from build123d import *

# Parameters (mm, degrees)
SKETCH_1_W                  = 720
SKETCH_1_H                  = 300
EXTRUDE_1_DEPTH             = 6
SKETCH_2_R                  = 30
CUT_EXTRUDE_1_DEPTH         = 13
SKETCH_5_R                  = 22.5
CUT_EXTRUDE_2_DEPTH         = 13
HOLE_WIZARD_M6_1_D          = 5
HOLE_WIZARD_13_0_13_1_D     = 13
HOLE_WIZARD_4_D             = 6.6
HOLE_WIZARD_4_CBORE_D       = 11
HOLE_WIZARD_4_CBORE_DEPTH   = 6.8
HOLE_WIZARD_11_0_11_1_D     = 11
HOLE_WIZARD_11_0_11_2_D     = 11
SKETCH_29_W                 = 170
SKETCH_29_H                 = 170
CUT_EXTRUDE_5_DEPTH         = 13
CUT_EXTRUDE_6_DEPTH         = 13
HOLE_WIZARD_M5_3_D          = 4.2
SKETCH_32_R                 = 28
CUT_EXTRUDE_7_DEPTH         = 13
HOLE_WIZARD_4_2_D           = 6.6
HOLE_WIZARD_4_2_CBORE_D     = 11
HOLE_WIZARD_4_2_CBORE_DEPTH = 6.8
HOLE_WIZARD_M6_2_D          = 5
SKETCH_38_W                 = 100
SKETCH_38_H                 = 110
CUT_EXTRUDE_8_DEPTH         = 13
HOLE_WIZARD_M6_3_D          = 5
FILLET_1_R                  = 10


with BuildPart() as part:
    # 草图1 → 凸台-拉伸1 (new body, symmetric)
    with BuildSketch(Plane.XY):
        Rectangle(SKETCH_1_W, SKETCH_1_H)
    extrude(amount=EXTRUDE_1_DEPTH, both=True)

    # 草图2 → 切除-拉伸1 (cut, through all)
    with BuildSketch(Plane.XY.offset(6)):
        with Locations((45, 0)):
            Circle(SKETCH_2_R)
    extrude(amount=-CUT_EXTRUDE_1_DEPTH, mode=Mode.SUBTRACT)

    # 草图5 → 切除-拉伸2 (cut, through all)
    with BuildSketch(Plane.XY.offset(6)):
        with Locations((-130, 87.5)):
            Circle(SKETCH_5_R)
        with Locations((-130, -87.5)):
            Circle(SKETCH_5_R)
        with Locations((220, -87.5)):
            Circle(SKETCH_5_R)
        with Locations((220, 87.5)):
            Circle(SKETCH_5_R)
    extrude(amount=-CUT_EXTRUDE_2_DEPTH, mode=Mode.SUBTRACT)

    # M6 螺纹孔1 (through all)
    with Locations(Plane.XY.offset(6)):
        with Locations((-154.5, -105), (-154.5, 105), (-105.5, 105), (-105.5, 70), (-154.5, 70), (244.5, 70), (195.5, 70), (195.5, 105), (244.5, 105), (244.5, -105), (195.5, -105), (195.5, -70), (244.5, -70), (-154.5, -70), (-105.5, -70), (-105.5, -105)):
            Hole(HOLE_WIZARD_M6_1_D / 2)

    # Ø13.0 (13) 直径孔1 (through all)
    with Locations(Plane.XY.offset(6)):
        with Locations((-65, 87.5), (155, 87.5), (155, -87.5), (-65, -87.5)):
            Hole(HOLE_WIZARD_13_0_13_1_D / 2)

    # Hole Wizard 4 (through all)
    with Locations(Plane(origin=(-240, 120, 6), x_dir=(1, 0, 0), z_dir=(0, 0, 1))):
        with Locations((0, 0), (40, 0), (40, -40), (0, -40), (40, -200), (40, -240), (0, -240), (0, -200), (530, 0), (570, 0), (570, -40), (530, -40), (530, -200), (570, -200), (570, -240), (530, -240)):
            CounterBoreHole(HOLE_WIZARD_4_D / 2, HOLE_WIZARD_4_CBORE_D / 2, HOLE_WIZARD_4_CBORE_DEPTH)

    # Ø11.0 (11) 直径孔1 (through all)
    with Locations(Plane(origin=(-30, 75, 6), x_dir=(1, 0, 0), z_dir=(0, 0, 1))):
        with Locations((0, 0), (152.597951226, 3.193252991), (0, -150), (150, -150)):
            Hole(HOLE_WIZARD_11_0_11_1_D / 2)

    # Ø11.0 (11) 直径孔2 (through all)
    with Locations(Plane(origin=(0.5, -44.5, 6), x_dir=(1, 0, 0), z_dir=(0, 0, 1))):
        with Locations((0, 0), (89, 0), (89, 89), (0, 89)):
            Hole(HOLE_WIZARD_11_0_11_2_D / 2)

    # 草图29 → 切除-拉伸5 (cut, through all)
    with BuildSketch(Plane.XY.offset(6)):
        with Locations((45, 0)):
            Rectangle(SKETCH_29_W, SKETCH_29_H)
    extrude(amount=-CUT_EXTRUDE_5_DEPTH, mode=Mode.SUBTRACT)

    # 草图30 → 切除-拉伸6 (cut, through all)
    with BuildSketch(Plane.XY.offset(6)):
        with BuildLine():
            Line((-90, 87.5), (-90, -87.5))
            ThreePointArc((-90, -87.5), (-130, -127.5), (-170, -87.5))
            Line((-170, -87.5), (-170, 87.5))
            ThreePointArc((-170, 87.5), (-130, 127.5), (-90, 87.5))
        make_face()
        with BuildLine():
            Line((260, 87.5), (260, -87.5))
            ThreePointArc((260, -87.5), (220, -127.5), (180, -87.5))
            Line((180, -87.5), (180, 87.5))
            ThreePointArc((180, 87.5), (220, 127.5), (260, 87.5))
        make_face()
    extrude(amount=-CUT_EXTRUDE_6_DEPTH, mode=Mode.SUBTRACT)

    # M5 螺纹孔3 (through all)
    with Locations(Plane(origin=(-336.75, 24.75, 6), x_dir=(1, 0, 0), z_dir=(0, 0, 1))):
        with Locations((0, 0), (49.5, 0), (49.5, -49.5), (0, -49.5)):
            Hole(HOLE_WIZARD_M5_3_D / 2)

    # 草图32 → 切除-拉伸7 (cut, through all)
    with BuildSketch(Plane.XY.offset(6)):
        with Locations((-312, 0)):
            Circle(SKETCH_32_R)
    extrude(amount=-CUT_EXTRUDE_7_DEPTH, mode=Mode.SUBTRACT)

    # Hole Wizard 4 2 (through all)
    with Locations(Plane(origin=(-353, -120, -6), x_dir=(-1, 0, 0), z_dir=(0, 0, -1))):
        with Locations((0, 0), (0, 120), (0, 240), (-53, 260), (-203, 260), (-353, 260), (-503, 260), (-653, 260), (-706, 240), (-706, 120), (-706, 0), (-653, -20), (-503, -20), (-353, -20), (-203, -20), (-53, -20)):
            CounterBoreHole(HOLE_WIZARD_4_2_D / 2, HOLE_WIZARD_4_2_CBORE_D / 2, HOLE_WIZARD_4_2_CBORE_DEPTH)

    # M6 螺纹孔2 (through all)
    with Locations(Plane(origin=(-341.8, 34.8, 6), x_dir=(1, 0, 0), z_dir=(0, 0, 1))):
        with Locations((0, 0), (69.6, 0), (69.6, -69.6), (0, -69.6)):
            Hole(HOLE_WIZARD_M6_2_D / 2)

    # 草图38 → 切除-拉伸8 (cut, through all)
    with BuildSketch(Plane.XY.offset(6)):
        with Locations((-295, 0)):
            Rectangle(SKETCH_38_W, SKETCH_38_H)
    extrude(amount=-CUT_EXTRUDE_8_DEPTH, mode=Mode.SUBTRACT)

    # M6 螺纹孔3 (through all)
    with Locations(Plane(origin=(-325, 65, 6), x_dir=(1, 0, 0), z_dir=(0, 0, 1))):
        with Locations((0, 0), (60, 0), (60, -130), (0, -130)):
            Hole(HOLE_WIZARD_M6_3_D / 2)

    # 圆角1
    fillet_1_edges = [part.edges().sort_by_distance(p)[0] for p in [
        (-245, 55, 0),
        (-245, -55, 0),
        (-345, -55, 0),
        (-345, 55, 0),
    ]]
    fillet(fillet_1_edges, radius=FILLET_1_R)


solid = part.part
For this review, take the finished solid that the model builds, in its own axes (mm). A direction names the side the tool comes from. Coordinates: 2 decimals unless noted, no trailing zeros. Order: outer loops, then holes, each group sorted by start corner. A loop starts at its lowest first (then second) coordinate and runs counter-clockwise, first axis right, second up. Notation, with made-up numbers: (21, 18.25) - (46, 18.25) arc R36 ccw to (46, 54.25) - close; hole circle Ø3 at (56, 4.5). An arc over 180 degrees is marked (long way). Answer as CSV lines item,"result". Start each with the question number.
1) Add section B-B (y = -18). State the section outline as (x, z) points, then the cut area to 3 significant figures.
2) Draft analysis for pull direction X (two halves, no side actions). For faces 3 (the flat face through (360, -2, 0)), 4 (the cylindrical face through (160.158, 83.545, -0.084)), 5 (the flat face through (-360, -2, 0)), state which applies: +X half, -X half, draft (parallel to the pull), parting line (faces both ways), or undercut.
3) Insertion check: P1, Ø14.5, axis at x = -200, y = 120, coming from the -Z side. The pin has a flat end and moves straight along its axis. Give the tip position at first contact, or say it passes through.
4) Add section D-D (x = 208.5). State the section outline as (y, z) points.
5) Add section C-C (y = -107). State the section outline as (x, z) points, then the cut area to 3 significant figures.
6) Machinability: for faces 1 (the flat face through (-170, -1, 0)), 2 (the flat face through (-5, -150, 0)), which of the approach directions +Z, -Z, +X, -X, +Y, -Y give a long, thin tool a straight path to every point of the face, cutting with its end or side? Answer none if there is none.
7) To check wall thickness, follow line 1 along X through (y, z) = (-58.5, -4.5); line 2 along X through (y, z) = (140, 2.6); line 3 along X through (y, z) = (-11, -3.25). State the ranges of each line that lie inside material, in increasing order. Write a range as [from, to].
8) Add section A-A (x = -65). State the section outline as (y, z) points, then the cut area to 3 significant figures.
Result:
1,outline,"(-360, -6) - (-345, -6) - (-345, 6) - (-360, 6) - close; (-245, -6) - (-170, -6) - (-170, 6) - (-245, 6) - close; (-90, -6) - (-40, -6) - (-40, 6) - (-90, 6) - close; (130, -6) - (180, -6) - (180, 6) - (130, 6) - close; (260, -6) - (360, -6) - (360, 6) - (260, 6) - close"
1,area,"3,480 mm^2"
2,face 3,"+X half"
2,face 4,"undercut"
2,face 5,"-X half"
3,P1,"z = -6"
4,outline,"(-150, -6) - (-125.81, -6) - (-125.81, 6) - (-150, 6) - close; (125.81, -6) - (150, -6) - (150, 6) - (125.81, 6) - close"
5,outline,"(-360, -6) - (-164.92, -6) - (-164.92, 6) - (-360, 6) - close; (-95.08, -6) - (185.08, -6) - (185.08, 6) - (-95.08, 6) - close; (254.92, -6) - (360, -6) - (360, 6) - (254.92, 6) - close"
5,area,"6,960 mm^2"
6,face 1,"+Z, -Z"
6,face 2,"+Z, -Z, +X, -X, -Y"
7,line 1,"[-360, -170], [-90, -40], [130, 180], [260, 360]"
7,line 2,"[-360, -303.3], [-296.7, -153.3], [-146.7, -3.3], [3.3, 146.7], [153.3, 296.7], [303.3, 360]"
7,line 3,"[-360, -345], [-245, -170], [-90, -40], [130, 180], [260, 360]"
8,outline,"(-150, -6) - (-94, -6) - (-94, 6) - (-150, 6) - close; (-81, -6) - (81, -6) - (81, 6) - (-81, 6) - close; (94, -6) - (150, -6) - (150, 6) - (94, 6) - close"
8,area,"3,290 mm^2"
